Could you check a few things on this model? Use its own coordinates, in mm. A direction names the side the tool comes from. Give positions to 0.01 mm unless a question says otherwise; leave off trailing zeros. Order: outer loops, then holes, each group sorted by start corner. A loop starts at its lowest first (then second) coordinate and runs counter-clockwise, first axis right, second up. Notation, with made-up numbers: (21.25, 28.25) - (40.25, 28.25) arc R18 cw to (40.25, 60.25) - close; hole circle Ø5 at (52.5, 9). An arc over 180 degrees is marked (long way). One line per question, with ' | ' between items. Start each with the question number.
1. If we mould it in two halves opening along X, with no side actions, what happens to faces 5 (the cylindrical face through (42, -3, 24)), 6 (the flat face through (-1, -6, -2)), 7 (the flat face through (-40.1, 3, 0)), 8 (the flat face through (-1, 4, 0))? For each: released by +X, released by -X, zero draft, split by the parting line, or undercut.
2. Imagine slicing it at B-B (x = -2.5). Please give me the cut outline in (y, z), and give its area (3 significant figures).
3. For P1, Ø9, axis at x = 6.5, y = 8, coming from the -Z side; P2, Ø2, axis at y = 7, z = 20.5, coming from the -X side; P3, Ø7.5, axis at y = 8, z = 17.5, coming from the +X side; P4, Ø1, axis at y = 0, z = -1, coming from the +X side, each with a flat end and sliding along its axis, tell me the tip position at first contact or that it passes through.
4. Which directions (+Z, -Z, +X, -X, +Y, -Y) give clear straight access to the entire face, cutting with the end or side of a thin tool? Please do faces 1 (the flat face through (30.1, 7, -19)), 2 (the flat face through (1, 3, -22.6)), 3 (the flat face through (-1, 3, 22.6)), 4 (the flat face through (-35, 7, -14.6)).
5. I need wall thicknesses on probe 1 along X at (y, z) = (8.5, 15); probe 2 along X at (y, z) = (2, -19); probe 3 along Z at (x, y) = (-12, 1). Which ranges of each line are inside material? Lowest first, please. Write a range as from..to.
6. Imagine slicing it at D-D (y = 2.25). Please give me the cut outline in (x, z), and give its area (3 significant figures).
7. Imagine slicing it at A-A (y = 7.75). Please give me the cut outline in (x, z), and give its area (3 significant figures).
8. Imagine slicing it at C-C (z = -20.5). Please give me the cut outline in (x, y).
```python
from build123d import *

# Parameters (mm, degrees)
PAD001_DEPTH = 6
PAD002_DEPTH = 4
SKETCH_W     = 10
SKETCH_H     = 8
PAD_DEPTH    = 7
FILLET_R     = 0.5


with BuildPart() as part:
    # Sketch008 → Pad001 (new body)
    with BuildSketch(Plane.XZ):
        with BuildLine():
            ThreePointArc((-40, 25), (-41.767767, 24.267767), (-42.5, 22.5))
            Line((-42.5, -27.5), (-42.5, 22.5))
            ThreePointArc((-42.5, -27.5), (-41.767767, -29.267767), (-40, -30))
            Line((40, -30), (-40, -30))
            ThreePointArc((40, -30), (41.767767, -29.267767), (42.5, -27.5))
            Line((42.5, 22.5), (42.5, -27.5))
            ThreePointArc((42.5, 22.5), (41.767767, 24.267767), (40, 25))
            Line((-40, 25), (40, 25))
        make_face()
    extrude(amount=PAD001_DEPTH)

    # Sketch009 → Pad002 (join)
    with BuildSketch(Plane.XZ):
        with BuildLine():
            ThreePointArc((-40, 22.6), (-40.070711, 22.570711), (-40.1, 22.5))
            Line((-40.1, -22.5), (-40.1, 22.5))
            ThreePointArc((-40.1, -22.5), (-40.070711, -22.570711), (-40, -22.6))
            Line((40, -22.6), (-40, -22.6))
            ThreePointArc((40, -22.6), (40.070711, -22.570711), (40.1, -22.5))
            Line((40.1, 22.5), (40.1, -22.5))
            ThreePointArc((40.1, 22.5), (40.070711, 22.570711), (40, 22.6))
            Line((-40, 22.6), (40, 22.6))
        make_face()
    extrude(amount=-PAD002_DEPTH)

    # Sketch → Pad (join)
    with BuildSketch(Plane.XZ.offset(-4)):
        with Locations((-35.1, 18.6)):
            Rectangle(SKETCH_W, SKETCH_H)
        with Locations((35.1, 18.6)):
            Rectangle(SKETCH_W, SKETCH_H)
        with Locations((35.1, -18.6)):
            Rectangle(SKETCH_W, SKETCH_H)
        with Locations((-35.1, -18.6)):
            Rectangle(SKETCH_W, SKETCH_H)
    extrude(amount=-PAD_DEPTH)

    # Fillet
    fillet_edges = [part.edges().sort_by_distance(p)[0] for p in [
        (-41.767767, -6, 24.267767),
        (0, -6, 25),
        (41.767767, -6, 24.267767),
        (42.5, -6, -2.5),
        (41.767767, -6, -29.267767),
        (0, -6, -30),
        (-41.767767, -6, -29.267767),
        (-42.5, -6, -2.5),
        (41.767767, 0, 24.267767),
        (0, 0, 25),
        (42.5, 0, -2.5),
        (41.767767, 0, -29.267767),
        (0, 0, -30),
        (-41.767767, 0, -29.267767),
        (-42.5, 0, -2.5),
        (-41.767767, 0, 24.267767),
    ]]
    fillet(fillet_edges, radius=FILLET_R)


solid = part.part
```
Results found:
1) face 5: released by +X | face 6: zero draft | face 7: released by -X | face 8: undercut
2) outline: (-6, -29.5) arc R0.5 ccw to (-5.5, -30) - (-0.5, -30) arc R0.5 ccw to (0, -29.5) - (0, -22.6) - (4, -22.6) - (4, 22.6) - (0, 22.6) - (0, 24.5) arc R0.5 ccw to (-0.5, 25) - (-5.5, 25) arc R0.5 ccw to (-6, 24.5) - close | area: 511 mm2
3) P1: stops at z = -22.6 | P2: stops at x = -40.1 | P3: stops at x = 40.1 | P4: stops at x = 42.5
4) face 1: +Z, -Z, +Y | face 2: -Z, +X, -X, +Y | face 3: +Z, +X, -X, +Y | face 4: +X, -X, +Y
5) probe 1: x = -40.1..-30.1, 30.1..40.1 | probe 2: x = -40.1..40.1 | probe 3: z = -22.6..22.6
6) outline: (-40.1, -22.5) arc R0.1 ccw to (-40, -22.6) - (40, -22.6) arc R0.1 ccw to (40.1, -22.5) - (40.1, 22.5) arc R0.1 ccw to (40, 22.6) - (-40, 22.6) arc R0.1 ccw to (-40.1, 22.5) - close | area: 3,630 mm2
7) outline: (-40.1, -22.6) - (-30.1, -22.6) - (-30.1, -14.6) - (-40.1, -14.6) - close; (-40.1, 14.6) - (-30.1, 14.6) - (-30.1, 22.6) - (-40.1, 22.6) - close; (30.1, -22.6) - (40.1, -22.6) - (40.1, -14.6) - (30.1, -14.6) - close; (30.1, 14.6) - (40.1, 14.6) - (40.1, 22.6) - (30.1, 22.6) - close | area: 320 mm2
8) outline: (-42.5, -5.5) arc R0.5 ccw to (-42, -6) - (42, -6) arc R0.5 ccw to (42.5, -5.5) - (42.5, -0.5) arc R0.5 ccw to (42, 0) - (40.1, 0) - (40.1, 11) - (30.1, 11) - (30.1, 4) - (-30.1, 4) - (-30.1, 11) - (-40.1, 11) - (-40.1, 0) - (-42, 0) arc R0.5 ccw to (-42.5, -0.5) - close
